Can you work these out from the model? Positions are in its coordinate system, mm. Face numbers are marked on the shaded views. A direction names the side the tool comes from. Round coordinates to 2 decimals unless told otherwise and drop trailing zeros. Loops run counter-clockwise (first coordinate to the right, second up) from the corner with the lowest first, then second, coordinate; pieces in that order, holes last. Notation, with made-up numbers: M -23.75,-32.5 L 9.25,-32.5 A18 ccw 9.25,-25.5 Z; hole C 60.25,-7 d8. An arc over 180 degrees is marked long. Answer as CSV lines item,"result".
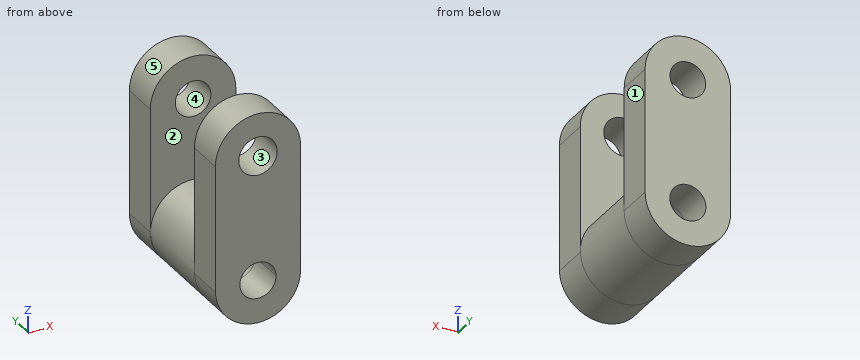
from build123d import *

# Parameters (mm, degrees)
F0_R     = 11.4715226447
F0_R_2   = 11.3474489307
F1_DEPTH = 25.4
F2_R     = 27.1514716213
F2_R_2   = 11.5339058998
F3_DEPTH = 53.34
F4_R     = 12.2446750111
F5_DEPTH = 25.4


with BuildPart() as f1:
    # F0 (on Front) → F1 (new body)
    with BuildSketch(Plane.XZ):
        with BuildLine():
            ThreePointArc((-27.219299227, -39.3772572279), (0, -12.1579580009), (27.219299227, -39.3772572279))
            Line((27.219299227, -39.3772572279), (27.219299227, 39.3772572279))
            ThreePointArc((27.219299227, 39.3772572279), (0, 12.1579580009), (-27.219299227, 39.3772572279))
            Line((-27.219299227, 39.3772572279), (-27.219299227, -39.3772572279))
        make_face()
        with BuildLine():
            ThreePointArc((-27.219299227, -39.3772572279), (0, -66.5965564549), (27.219299227, -39.3772572279))
            ThreePointArc((27.219299227, -39.3772572279), (0, -12.1579580009), (-27.219299227, -39.3772572279))
        make_face()
        with Locations((0, -39.3772572279)):
            Circle(F0_R, mode=Mode.SUBTRACT)
        with BuildLine():
            ThreePointArc((-27.219299227, 39.3772572279), (0, 12.1579580009), (27.219299227, 39.3772572279))
            ThreePointArc((27.219299227, 39.3772572279), (0, 66.5965564549), (-27.219299227, 39.3772572279))
        make_face()
        with Locations((0, 39.3772572279)):
            Circle(F0_R_2, mode=Mode.SUBTRACT)
    extrude(amount=F1_DEPTH)

    # F2 (on face) → F3 (join)
    with BuildSketch(Plane.XZ.offset(25.4)):
        with Locations((0, -39.3772572279)):
            Circle(F2_R)
        with Locations((0, -39.3772572279)):
            Circle(F2_R_2, mode=Mode.SUBTRACT)
    extrude(amount=F3_DEPTH)

    # F4 (on face) → F5 (join)
    with BuildSketch(Plane.XZ.offset(78.74)):
        with BuildLine():
            ThreePointArc((-27.1369592055, -40.2648699161), (0, -66.5287288492), (27.1369592055, -40.2648699161))
            Line((27.1369592055, -40.2648699161), (27.1369592055, -38.4896445397))
            ThreePointArc((27.1369592055, -38.4896445397), (0, -12.2257856066), (-27.1369592055, -38.4896445397))
            Line((-27.1369592055, -38.4896445397), (-27.1369592055, -40.2648699161))
        make_face()
        with BuildLine():
            ThreePointArc((4.719235111, -28.8530087858), (10.2659715637, -33.4010821613), (12.3491600723, -40.2648699161))
            ThreePointArc((12.3491600723, -40.2648699161), (-6.8637877548, -50.5308414798), (-4.719235111, -28.8530087858))
            ThreePointArc((-4.719235111, -28.8530087858), (0, -27.8433513281), (4.719235111, -28.8530087858))
        make_face(mode=Mode.SUBTRACT)
        with BuildLine():
            ThreePointArc((-27.1369592055, -38.4896445397), (0, -12.2257856066), (27.1369592055, -38.4896445397))
            Line((27.1369592055, -38.4896445397), (27.1369592055, 40.2648699161))
            ThreePointArc((27.1369592055, 40.2648699161), (0, 13.1279107106), (-27.1369592055, 40.2648699161))
            Line((-27.1369592055, 40.2648699161), (-27.1369592055, -38.4896445397))
        make_face()
        with BuildLine():
            ThreePointArc((-27.1369592055, 40.2648699161), (0, 13.1279107106), (27.1369592055, 40.2648699161))
            ThreePointArc((27.1369592055, 40.2648699161), (0, 67.4018291216), (-27.1369592055, 40.2648699161))
        make_face()
        with Locations((0, 40.2648699161)):
            Circle(F4_R, mode=Mode.SUBTRACT)
        with BuildLine():
            ThreePointArc((-4.719235111, -28.8530087858), (-6.8637877548, -50.5308414798), (12.3491600723, -40.2648699161))
            ThreePointArc((12.3491600723, -40.2648699161), (10.2659715637, -33.4010821613), (4.719235111, -28.8530087858))
            ThreePointArc((4.719235111, -28.8530087858), (9.6814822985, -33.1082951282), (11.5339058998, -39.3772572279))
            ThreePointArc((11.5339058998, -39.3772572279), (-6.2689620997, -49.0587395264), (-4.719235111, -28.8530087858))
        make_face()
    extrude(amount=F5_DEPTH)


solid = f1.part
Item 1: Will these pins go through, and if not, where does the flat tip stop? pin 1 (12.5 mm diameter, centred on y = -94.5, z = -16.5, fed in from -X); pin 2 (12.5 mm diameter, centred on y = -95, z = -2.5, fed in from +X); pin 3 (14 mm diameter, centred on x = 0, z = -39.38, fed in from -Y); pin 4 (3 mm diameter, centred on x = 1.5, y = -29.5, fed in from +Z).
Output:
pin 1,"stops at x = -27.14"
pin 2,"stops at x = 27.14"
pin 3,"passes through"
pin 4,"stops at z = -12.23"
Item 2: If we section it at C-C on y = -22: Write out the boundary of the cut face in (x, z).
Output:
outline,"M -27.22,-39.38 A27.22 ccw 27.22,-39.38 L 27.22,39.38 A27.22 ccw -27.22,39.38 Z; hole C 0,-39.38 d22.94; hole C 0,39.38 d22.69"
Item 3: On a 3-axis mill with a long thin cutter (end or side, diameter ignored), from which of +Z, -Z, +X, -X, +Y, -Y can I reach the whole of each face in a straight line? I mean the marked faces 4 and 5. Say none if no direction works.
Output:
face 4,"+Y, -Y"
face 5,"+Z, +Y"
Item 4: We'd pull the mould along X, two halves only. Please class the marked faces 1, 2 and 3: released by +X, released by -X, zero draft, split by the parting line, or undercut.
Output:
face 1,"released by +X"
face 2,"zero draft"
face 3,"undercut"
Item 5: If we section it at B-B on z = 36: Write out the boundary of the cut face in (x, y), then the cut area to 3 significant figures.
Output:
outline,"M -27.22,-25.4 L -10.83,-25.4 L -10.83,0 L -27.22,0 Z; M -27.14,-104.14 L -11.48,-104.14 L -11.48,-78.74 L -27.14,-78.74 Z; M 10.83,-25.4 L 27.22,-25.4 L 27.22,0 L 10.83,0 Z; M 11.48,-104.14 L 27.14,-104.14 L 27.14,-78.74 L 11.48,-78.74 Z"
area,"1,630 mm2"
Item 6: If I drill on line 1 along Z through (x, y) = (0, -13); line 2 along Y through (x, z) = (8, 9); line 3 along Z through (x, y) = (0.5, -54), over which ranges is the centre line in solid material (lowest first)? Write a range as from..to.
Output:
line 1,"z = -66.6..-50.85, -27.91..28.03, 50.72..66.6"
line 2,"y = -104.14..-78.74, -25.4..0"
line 3,"z = -66.52..-50.9, -27.85..-12.23"
Item 7: If we section it at D-D on y = -53.5: Write out the boundary of the cut face in (x, z), then the cut area to 3 significant figures.
Output:
outline,"C 0,-39.38 d54.3; hole C 0,-39.38 d23.07"
area,"1,900 mm2"
Item 8: If we section it at A-A on x = 0: Write out the boundary of the cut face in (y, z), then the cut area to 3 significant figures.
Output:
outline,"M -104.14,-66.53 L -25.4,-66.53 L -25.4,-66.6 L 0,-66.6 L 0,-50.85 L -25.4,-50.85 L -25.4,-50.91 L -104.14,-50.91 Z; M -104.14,-27.84 L -25.4,-27.84 L -25.4,-27.91 L 0,-27.91 L 0,28.03 L -25.4,28.03 L -25.4,-12.23 L -78.74,-12.23 L -78.74,28.02 L -104.14,28.02 Z; M -104.14,52.51 L -78.74,52.51 L -78.74,67.4 L -104.14,67.4 Z; M -25.4,50.72 L 0,50.72 L 0,66.6 L -25.4,66.6 Z"
area,"6,080 mm2"
